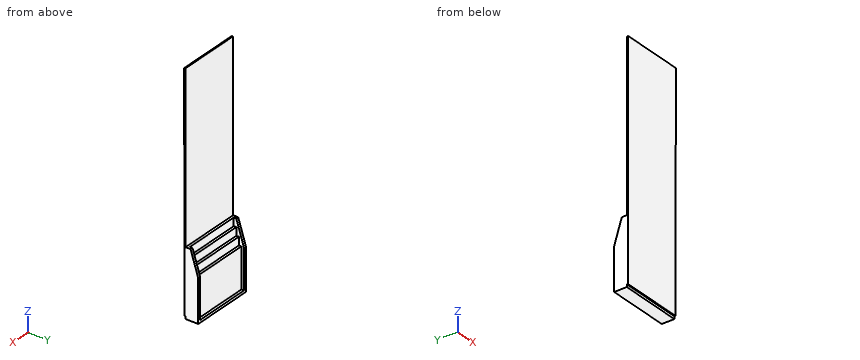
```python
from build123d import *

# Parameters (mm, degrees)
BOSS_EXTRUDE1_DEPTH = 500
BOSS_EXTRUDE2_DEPTH = 22
LPATTERN1_COUNT     = 2
LPATTERN1_PITCH     = 522
SKETCH3_W           = 22
SKETCH3_H           = 110
BOSS_EXTRUDE3_DEPTH = 500
SKETCH4_W           = 544
SKETCH4_H           = 2000
BOSS_EXTRUDE4_DEPTH = 10


with BuildPart() as part:
    # Sketch1 → Boss-Extrude1 (new body)
    with BuildSketch(Plane(origin=(0, 0, 0), x_dir=(0, 0, -1), z_dir=(1, 0, 0))):
        Polygon((1.256226638, 87.216565021), (349.256226638, 87.216565021), (349.256226638, 0), (-208.743773362, -0.783434979), (-208.743773362, 21.216565021), (-138.743773362, 21.216565021), (-138.743773362, 43.216565021), (-68.743773362, 43.216565021), (-68.743773362, 65.216565021), (1.256226638, 65.216565021), align=None)
    extrude(amount=BOSS_EXTRUDE1_DEPTH)

    # Sketch2 → Boss-Extrude2 (add)
    with BuildSketch(Plane(origin=(500, 0, 0), x_dir=(0, 0, -1), z_dir=(1, 0, 0))):
        Polygon((-208.743773362, -0.783434979), (-208.743773362, 43.216565021), (1.256226638, 110), (371.256226638, 110), (371.256226638, 0), (349.256226638, 0), align=None)
    boss_extrude2 = extrude(amount=BOSS_EXTRUDE2_DEPTH)

    # LPattern1: Boss-Extrude2 ×2
    with Locations(*[(-i * LPATTERN1_PITCH, 0, 0) for i in range(1, LPATTERN1_COUNT)]):
        add(boss_extrude2)

    # Sketch3 → Boss-Extrude3 (add)
    with BuildSketch(Plane(origin=(0, 0, 0), x_dir=(0, 0, -1), z_dir=(1, 0, 0))):
        with Locations((360.256226638, 55)):
            Rectangle(SKETCH3_W, SKETCH3_H)
    extrude(amount=BOSS_EXTRUDE3_DEPTH)

    # Sketch4 → Boss-Extrude4 (add)
    with BuildSketch(Plane(origin=(0, -0.49035664, -0.000688463), x_dir=(1, 0, 0), z_dir=(0, -0.9999990143859607, -0.0014040039555169115))):
        with Locations((250, 650.744117594)):
            Rectangle(SKETCH4_W, SKETCH4_H)
    extrude(amount=BOSS_EXTRUDE4_DEPTH)


solid = part.part
```
Geometry check sheet. Reference: the model listing, model coordinates, mm. Give positions to 0.01 mm unless a question says otherwise; leave off trailing zeros. Order: outer loops, then holes, each group sorted by start corner. A loop starts at its lowest first (then second) coordinate and runs counter-clockwise, first axis right, second up. Notation, with made-up numbers: (81, -27.5) - (110, -27.5) arc R27 ccw to (110, -11.5) - close; hole circle Ø6 at (25, 63). An arc over 180 degrees is marked (long way). Answer in a Markdown table with one row per item. Add a question column.
Q1. Cross-section at B-B, the plane z = 928. Enter the section's corners in (x, y), then the cut area to 3 significant figures.
Q2. Cross-section at A-A, the plane x = 186. Enter the section's corners in (y, z).
Q3. Material ranges on probe 1 along X at (y, z) = (88, -224.5); probe 2 along Z at (x, y) = (267.5, 61); probe 3 along Z at (x, y) = (20, 78.5), recorded low to high. Write a range as from..to.
Q4. Gauge pin test, flat ends, axial feed: pin 1 (1.5 mm diameter, centred on x = 281.5, z = 311, fed in from +Y); pin 2 (12 mm diameter, centred on x = 430, y = 21, fed in from +Z); pin 3 (11 mm diameter, centred on x = 161, y = 77, fed in from +Z). Record the tip position at first contact, or that the pin passes through.
Check values:
| question | item | result |
|---|---|---|
| 1 | outline | (-22, -11.79) - (522, -11.79) - (522, -1.79) - (-22, -1.79) - close |
| 1 | area | 5,440 mm^2 |
| 2 | outline | (-12.81, 1650.73) - (-10, -349.27) - (0, -349.26) - (0, -371.26) - (110, -371.26) - (110, -349.26) - (87.22, -349.26) - (87.22, -1.26) - (65.22, -1.26) - (65.22, 68.74) - (43.22, 68.74) - (43.22, 138.74) - (21.22, 138.74) - (21.22, 208.74) - (-0.78, 208.74) - (-2.81, 1650.74) - close |
| 3 | probe 1 | x = -22..0, 500..522 |
| 3 | probe 2 | z = -371.26..68.74 |
| 3 | probe 3 | z = -371.26..-1.26 |
| 4 | pin 1 | stops at y = -0.93 |
| 4 | pin 2 | stops at z = 208.74 |
| 4 | pin 3 | stops at z = -1.26 |
